The listing builds one solid part. Answer for the finished solid, in the listing's coordinates (mm). Face numbers are marked on the shaded views. A direction names the side the tool comes from. Give positions to 0.01 mm unless a question says otherwise; leave off trailing zeros. Write each loop counter-clockwise with the first axis right and the second up, starting at its lowest first coordinate (ties: lowest second). Pieces come first, ordered by that corner, then holes. Notation, with made-up numbers: M -5.75,20 L 5.25,20 A13 ccw 5.25,45 Z; hole C 28,82.25 d6. An arc over 180 degrees is marked long. Return JSON: item names as keys, results as strings.
from build123d import *

# Parameters (mm, degrees)
SKETCH_1_R      = 1.55
EXTRUDE_1_DEPTH = 27.5


with BuildPart() as part:
    # 草图1 → 凸台-拉伸1 (new body)
    with BuildSketch(Plane.XY):
        with BuildLine():
            Line((2.165063509, 1.25), (14, 1.25))
            Line((14, 1.25), (14, -0.45))
            Line((14, -0.45), (11.014359354, -1.25))
            Line((11.014359354, -1.25), (2.165063509, -1.25))
            ThreePointArc((2.165063509, -1.25), (0, -2.5), (-2.165063509, -1.25))
            Line((-2.165063509, -1.25), (-14, -1.25))
            Line((-14, -1.25), (-14, 0.25))
            ThreePointArc((-14, 0.25), (-13.707106781, 0.957106781), (-13, 1.25))
            Line((-13, 1.25), (-2.165063509, 1.25))
            ThreePointArc((-2.165063509, 1.25), (0, 2.5), (2.165063509, 1.25))
        make_face()
        Circle(SKETCH_1_R, mode=Mode.SUBTRACT)
    extrude(amount=EXTRUDE_1_DEPTH)


solid = part.part
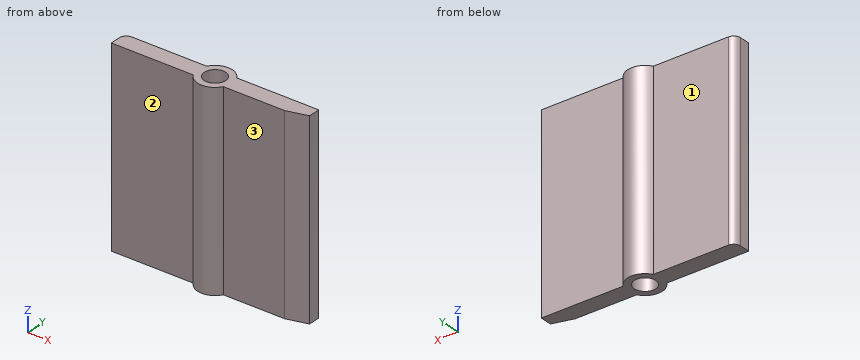
Item 1: Find the intervals of material crossed by line 1 (X direction, y = 1.15, z = 9.5); line 2 (Y direction, x = 3, z = 18.75); line 3 (X direction, y = 0.55, z = 14), in increasing order.
Geometry results:
{"line 1": "x = -13.44 to -1.04, 1.04 to 14", "line 2": "y = -1.25 to 1.25", "line 3": "x = -13.95 to -1.45, 1.45 to 14"}
Item 2: A cutting plane is placed at A-A, the plane z = 12.25. Write down the section's boundary in (x, y).
Geometry results:
{"outline": "M -14,-1.25 L -2.17,-1.25 A2.5 ccw 2.17,-1.25 L 11.01,-1.25 L 14,-0.45 L 14,1.25 L 2.17,1.25 A2.5 ccw -2.17,1.25 L -13,1.25 A1 ccw -14,0.25 Z; hole C 0,0 d3.1"}
Item 3: A cutting plane is placed at B-B, the plane x = 0. Write down the section's boundary in (y, z).
Geometry results:
{"outline": "M -2.5,0 L -1.55,0 L -1.55,27.5 L -2.5,27.5 Z; M 1.55,0 L 2.5,0 L 2.5,27.5 L 1.55,27.5 Z"}
Item 4: Given pin 1 Ø12 at (x, z) = (-9.5, 9.5) entering from +Y; pin 2 Ø2 at (x, y) = (4, 0) entering from -Z; pin 3 Ø7 at (x, z) = (5, 15.5) entering from -Y; pin 4 Ø6 at (x, z) = (-6, 11.5) entering from -Y, each flat-ended and moving along its own axis, determine where each tip first touches the part or whether it passes through.
Geometry results:
{"pin 1": "stops at y = 1.25", "pin 2": "stops at z = 0", "pin 3": "stops at y = -2", "pin 4": "stops at y = -1.25"}
Item 5: A cutting plane is placed at D-D, the plane x = -4.25. Write down the section's boundary in (y, z), plus the area to 4 significant figures.
Geometry results:
{"outline": "M -1.25,0 L 1.25,0 L 1.25,27.5 L -1.25,27.5 Z", "area": "68.75 mm2"}
Item 6: A cutting plane is placed at C-C, the plane y = 0.85. Write down the section's boundary in (x, z), plus the area to 3 significant figures.
Geometry results:
{"outline": "M -13.8,0 L -1.3,0 L -1.3,27.5 L -13.8,27.5 Z; M 1.3,0 L 14,0 L 14,27.5 L 1.3,27.5 Z", "area": "693 mm2"}
Item 7: Which of the six approach directions +Z, -Z, +X, -X, +Y, -Y give full straight-line access (tool end or side, diameter ignored) to the marked faces 1, 2 and 3?
Geometry results:
{"face 1": "+Z, -Z, -X, +Y", "face 2": "+Z, -Z, -X, -Y", "face 3": "+Z, -Z, +X, -Y"}
